```python
from build123d import *
from OCP.BRepFilletAPI import BRepFilletAPI_MakeChamfer

# Parameters (mm, degrees)
SKETCH1_W                        = 101.6
SKETCH1_H                        = 76.2
EXTRUDE1_DEPTH                   = 76.2
EXTRUDE2_DEPTH                   = 6.35
F_10_24_TAPPED_HOLE1_D           = 3.7973
F_10_24_TAPPED_HOLE1_DEPTH       = 12.954
F_10_24_TAPPED_HOLE1_TIP         = 1.140824014
EXTRUDE3_DEPTH                   = 6.35
CHAMFER1_SIZE                    = 6.35
CHAMFER1_SIZE2                   = 6.479869459
EXTRUDE4_DEPTH                   = 6.35
SKETCH8_W                        = 101.6
SKETCH8_H                        = 76.2
EXTRUDE5_DEPTH                   = 2.54
F_10_24_TAPPED_HOLE2_D           = 3.7973
F_10_24_TAPPED_HOLE2_DEPTH       = 12.954
F_10_24_TAPPED_HOLE2_CBORE_D     = 4.826
F_10_24_TAPPED_HOLE2_CBORE_DEPTH = 9.652
F_10_24_TAPPED_HOLE2_TIP         = 1.140824014


with BuildPart() as part:
    # Sketch1 → Extrude1 (new body)
    with BuildSketch(Plane(origin=(0, 0, 0), x_dir=(1, 0, 0), z_dir=(0, 1, 0))):
        with Locations((50.8, 38.1)):
            Rectangle(SKETCH1_W, SKETCH1_H)
    extrude(amount=-EXTRUDE1_DEPTH)

    # Sketch3 → Extrude2 (add)
    with BuildSketch(Plane.XY):
        with BuildLine():
            Line((19.05, -4.754440133), (82.55, -4.754440133))
            ThreePointArc((82.55, -4.754440133), (89.285192091, -7.544248042), (92.075, -14.279440133))
            Line((92.075, -14.279440133), (92.075, -52.379440133))
            ThreePointArc((92.075, -52.379440133), (89.285192091, -59.114632223), (82.55, -61.904440133))
            Line((82.55, -61.904440133), (19.05, -61.904440133))
            ThreePointArc((19.05, -61.904440133), (12.314807909, -59.114632223), (9.525, -52.379440133))
            Line((9.525, -52.379440133), (9.525, -14.279440133))
            ThreePointArc((9.525, -14.279440133), (12.314807909, -7.544248042), (19.05, -4.754440133))
        make_face()
        with BuildLine():
            Line((19.05, -11.104440133), (82.55, -11.104440133))
            ThreePointArc((82.55, -11.104440133), (84.79506403, -12.034376102), (85.725, -14.279440133))
            Line((85.725, -14.279440133), (85.725, -52.379440133))
            ThreePointArc((85.725, -52.379440133), (84.79506403, -54.624504163), (82.55, -55.554440133))
            Line((82.55, -55.554440133), (19.05, -55.554440133))
            ThreePointArc((19.05, -55.554440133), (16.80493597, -54.624504163), (15.875, -52.379440133))
            Line((15.875, -52.379440133), (15.875, -14.279440133))
            ThreePointArc((15.875, -14.279440133), (16.80493597, -12.034376102), (19.05, -11.104440133))
        make_face(mode=Mode.SUBTRACT)
    extrude(amount=EXTRUDE2_DEPTH)

    # #10-24 Tapped Hole1
    with Locations(Plane(origin=(12.7, -33.329440133, 6.35), x_dir=(1, 0, 0), z_dir=(0, 0, 1))):
        with Locations((0, 0), (76.2, 0)):
            Hole(F_10_24_TAPPED_HOLE1_D / 2, depth=F_10_24_TAPPED_HOLE1_DEPTH)
            with Locations((0, 0, -(F_10_24_TAPPED_HOLE1_DEPTH + F_10_24_TAPPED_HOLE1_TIP / 2))):  # 118° drill point
                Cone(0, F_10_24_TAPPED_HOLE1_D / 2, F_10_24_TAPPED_HOLE1_TIP, mode=Mode.SUBTRACT)

    # Sketch6 → Extrude3 (add)
    with BuildSketch(Plane.XY):
        Polygon((82.55, -4.754440133), (91.885938624, -4.754440133), (92.075, -14.279440133), align=None)
        Polygon((92.075, -52.379440133), (82.55, -61.904440133), (92.075, -61.904440133), align=None)
        Polygon((9.525, -14.279440133), (19.05, -4.754440133), (9.525, -4.754440133), align=None)
        Polygon((9.525, -52.379440133), (19.05, -61.904440133), (9.525, -61.904440133), align=None)
    extrude(amount=EXTRUDE3_DEPTH)

    # Chamfer1: one chamfer whose edges measure the first distance from different faces: ONE call of the kernel's chamfer builder (chamfer() names one face for all edges)
    chamfer1_edges_1 = [part.edges().sort_by_distance(p)[0] for p in [
        (92.075, -61.904440133, 3.175),
        (9.525, -61.904440133, 3.175),
        (9.525, -4.754440133, 3.175),
    ]]
    chamfer1_edges_2 = [part.edges().sort_by_distance(p)[0] for p in [
        (91.885938624, -4.754440133, 3.175),
    ]]
    chamfer1_side_2 = [part.faces().sort_by_distance(p)[0] for p in [
        (91.976718118, -9.327953214, 3.175),
    ]]
    chamfer1 = BRepFilletAPI_MakeChamfer(part.part.solid().wrapped)
    for e in chamfer1_edges_1:
        chamfer1.Add(CHAMFER1_SIZE, e.wrapped)
    for e in chamfer1_edges_2:
        chamfer1.Add(CHAMFER1_SIZE, CHAMFER1_SIZE2, e.wrapped, chamfer1_side_2[0].wrapped)  # the first distance lies on this face
    add(Compound.cast(chamfer1.Shape()), mode=Mode.REPLACE)



with BuildPart() as body_2:
    # Sketch7 → Extrude4 (new body)
    with BuildSketch(Plane(origin=(0, 0, -78.74), x_dir=(-1, 0, 0), z_dir=(0, 0, -1))):
        Polygon((-85.406069165, -4.754440133), (-15.875, -4.754440133), (-9.525, -11.104440133), (-9.525, -55.554440133), (-15.875, -61.904440133), (-85.725, -61.904440133), (-92.075, -55.554440133), (-92.075, -11.103141464), align=None)
        with BuildLine():
            Line((-15.875, -14.406440133), (-15.875, -52.252440133))
            ThreePointArc((-15.875, -52.252440133), (-16.842133409, -54.587306724), (-19.177, -55.554440133))
            Line((-19.177, -55.554440133), (-82.423, -55.554440133))
            ThreePointArc((-82.423, -55.554440133), (-84.757866591, -54.587306724), (-85.725, -52.252440133))
            Line((-85.725, -52.252440133), (-85.725, -14.406440133))
            ThreePointArc((-85.725, -14.406440133), (-84.757866591, -12.071573541), (-82.423, -11.104440133))
            Line((-82.423, -11.104440133), (-19.177, -11.104440133))
            ThreePointArc((-19.177, -11.104440133), (-16.842133409, -12.071573541), (-15.875, -14.406440133))
        make_face(mode=Mode.SUBTRACT)
    extrude(amount=EXTRUDE4_DEPTH)


with BuildPart() as part_1:
    add(part.part)

    add(body_2.part)  # Extrude5 merges body 2
    # Sketch8 → Extrude5 (add)
    with BuildSketch(Plane(origin=(0, 0, -76.2), x_dir=(-1, 0, 0), z_dir=(0, 0, -1))):
        with Locations((-50.8, -38.1)):
            Rectangle(SKETCH8_W, SKETCH8_H)
    extrude(amount=EXTRUDE5_DEPTH)

    # #10-24 Tapped Hole2
    with Locations(Plane(origin=(88.9, -33.329440133, -85.09), x_dir=(-1, 0, 0), z_dir=(0, 0, -1))):
        with Locations((0, 0), (76.2, 0)):
            CounterBoreHole(F_10_24_TAPPED_HOLE2_D / 2, F_10_24_TAPPED_HOLE2_CBORE_D / 2, F_10_24_TAPPED_HOLE2_CBORE_DEPTH, depth=F_10_24_TAPPED_HOLE2_DEPTH)
            with Locations((0, 0, -(F_10_24_TAPPED_HOLE2_DEPTH + F_10_24_TAPPED_HOLE2_TIP / 2))):  # 118° drill point
                Cone(0, F_10_24_TAPPED_HOLE2_D / 2, F_10_24_TAPPED_HOLE2_TIP, mode=Mode.SUBTRACT)


solid = part_1.part
```
Model file for the job. Use its own axes, mm. A direction names the side the tool comes from. Give positions to 0.01 mm unless a question says otherwise; leave off trailing zeros. Loops run counter-clockwise (first coordinate to the right, second up) from the corner with the lowest first, then second, coordinate; pieces in that order, holes last. Notation, with made-up numbers: (-20, -6.75) - (4, -6.75) arc R6 ccw to (4, 0.25) - close; hole circle Ø3 at (28.25, -13). An arc over 180 degrees is marked (long way). One line per item, written item: value. Start each with the question number.
1. Slice it at C-C (x = 95). List the corners of the cut face in (y, z).
2. Slice it at A-A (y = -22.5). List the corners of the cut face in (x, z) (3 decimals), plus the area to 3 significant figures.
3. Probe L1, parallel to Y at x = 88.9, z = -73.9; L2, parallel to Z at x = 90, y = -4.5; L3, parallel to Y at x = 36, z = 3. List the from-to ranges inside material, lowest first. Write a range as from..to.
4. Which spindle directions (+Z, -Z, +X, -X, +Y, -Y) get a long thin tool onto all of the face, cutting with end or side? Do faces 5 (the flat face through (51, -11.104, -82)), 6 (the flat face through (88.787, -7.973, -81.871)), 7 (the flat face through (50, -11.104, 3)), 8 (the flat face through (88.86, -58.77, -81.87)). Say none if no direction does.
5. Pin check, flat tips, straight feed: pin 1 (6 mm diameter, centred on y = -29, z = -3, fed in from -X); pin 2 (1.5 mm diameter, centred on x = 74.5, y = -49, fed in from +Z); pin 3 (5 mm diameter, centred on y = -24.5, z = -83.5, fed in from +X) (3 decimals); pin 4 (4.5 mm diameter, centred on x = 88.9, y = -33.33, fed in from -Z). Stop position of each tip, or through.
6. Pull direction X, two halves, no side cores. Call faces 1 (the flat face through (92.075, -35, 3)), 2 (the cylindrical face through (89.8, -35, -73.8)), 3 (the flat face through (51, -33, -78.74)), 4 (the flat face through (51, -61.904, 3)): pulls with the +X half, pulls with the -X half, needs draft (parallel to the pull), parting line crosses it, or undercut.
7. Slice it at B-B (x = 21). List the corners of the cut face in (y, z).
Solution:
1. outline: (-76.2, -78.74) - (0, -78.74) - (0, 0) - (-76.2, 0) - close
2. outline: (0, -78.74) - (9.525, -78.74) - (9.525, -85.09) - (15.875, -85.09) - (15.875, -78.74) - (85.725, -78.74) - (85.725, -85.09) - (92.075, -85.09) - (92.075, -78.74) - (101.6, -78.74) - (101.6, 0) - (92.075, 0) - (92.075, 6.35) - (85.725, 6.35) - (85.725, 0) - (15.875, 0) - (15.875, 6.35) - (9.525, 6.35) - (9.525, 0) - (0, 0) - close
2. area: 8,160 mm^2
3. L1: y = -76.2..-35.23, -31.43..0
3. L2: z = -78.74..0
3. L3: y = -61.9..-55.55, -11.1..-4.75
4. face 5: -Z
4. face 6: -Z, +X, +Y
4. face 7: +Z
4. face 8: -Z, +X, -Y
5. pin 1: stops at x = 0
5. pin 2: stops at z = 0
5. pin 3: stops at x = 92.075
5. pin 4: stops at z = -75.44
6. face 1: pulls with the +X half
6. face 2: undercut
6. face 3: undercut
6. face 4: needs draft
7. outline: (-76.2, -78.74) - (-61.9, -78.74) - (-61.9, -85.09) - (-55.55, -85.09) - (-55.55, -78.74) - (-11.1, -78.74) - (-11.1, -85.09) - (-4.75, -85.09) - (-4.75, -78.74) - (0, -78.74) - (0, 0) - (-4.75, 0) - (-4.75, 6.35) - (-11.1, 6.35) - (-11.1, 0) - (-55.55, 0) - (-55.55, 6.35) - (-61.9, 6.35) - (-61.9, 0) - (-76.2, 0) - close
